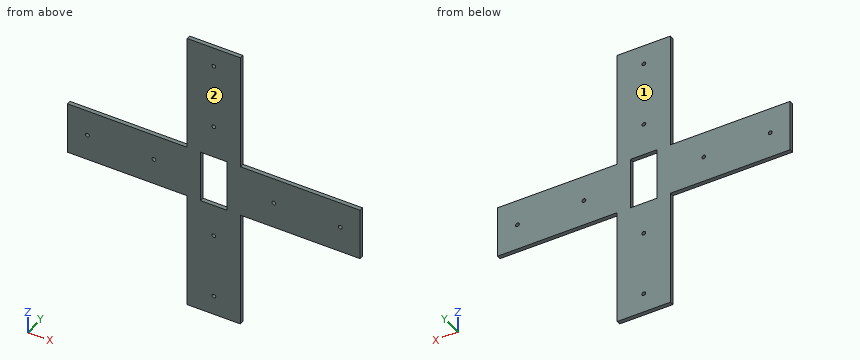
```python
from build123d import *

# Parameters (mm, degrees)
SKETCH1_R           = 1.45
SKETCH1_W           = 20.1
SKETCH1_H           = 40.1
BOSS_EXTRUDE1_DEPTH = 3


with BuildPart() as part:
    # Sketch1 → Boss-Extrude1 (new body)
    with BuildSketch(Plane(origin=(0, 0, 0), x_dir=(1, 0, 0), z_dir=(0, 1, 0))):
        Polygon((-20, 110), (20, 110), (20, 20), (110, 20), (110, -20), (20, -20), (20, -110), (-20, -110), (-20, -20), (-110, -20), (-110, 20), (-20, 20), align=None)
        with Locations(Location((45, 0, 0), (0, 0, 270))):
            Circle(SKETCH1_R, mode=Mode.SUBTRACT)
        with Locations(Location((95, 0, 0), (0, 0, 270))):
            Circle(SKETCH1_R, mode=Mode.SUBTRACT)
        with Locations(Location((-95, 0, 0), (0, 0, 270))):
            Circle(SKETCH1_R, mode=Mode.SUBTRACT)
        with Locations(Location((-45, 0, 0), (0, 0, 270))):
            Circle(SKETCH1_R, mode=Mode.SUBTRACT)
        with Locations(Location((0, 95, 0), (0, 0, 270))):
            Circle(SKETCH1_R, mode=Mode.SUBTRACT)
        with Locations(Location((0, 45, 0), (0, 0, 270))):
            Circle(SKETCH1_R, mode=Mode.SUBTRACT)
        with Locations(Location((0, -45, 0), (0, 0, 270))):
            Circle(SKETCH1_R, mode=Mode.SUBTRACT)
        with Locations(Location((0, -95, 0), (0, 0, 270))):
            Circle(SKETCH1_R, mode=Mode.SUBTRACT)
        Rectangle(SKETCH1_W, SKETCH1_H, mode=Mode.SUBTRACT)
    extrude(amount=BOSS_EXTRUDE1_DEPTH)


solid = part.part
```
Source: CAD feature listing. Evaluate the final solid. Frame: model axes, mm. Face numbers are marked on the shaded views. Give positions to 0.01 mm unless a question says otherwise; leave off trailing zeros. Order: outer loops, then holes, each group sorted by start corner. A loop starts at its lowest first (then second) coordinate and runs counter-clockwise, first axis right, second up.
(1) Section query A-A (y = 0.45). State how many separate pieces and enclosed holes the cut face has, plus the area to 3 significant figures.
(2) Material intervals for line 1 along X through (y, z) = (2.1, 0); line 2 along X through (y, z) = (1.85, 45), sorted ascending.
(3) Section query B-B (z = -52.5). Return the cut outline in (x, y).
(4) Pull-direction query (Y, two-part tool) for the marked faces 1 and 2; classes: +Y half, -Y half, draft (parallel to the pull), parting line (faces both ways), or undercut.
(5) Contact query for flat-ended pins moving along their axis: P1, Ø4.5, axis at x = 0, z = -45, coming from the +Y side; P2, Ø1.5, axis at y = 1.5, z = -86.5, coming from the -X side; P3, Ø0.9, axis at x = 53.5, y = 2, coming from the -Z side. Output: stop coordinate, or through.
(6) Section query C-C (x = -34). Return the cut outline in (y, z), plus the area to 3 significant figures.
Outcome:
1. separate pieces: 1
1. enclosed holes: 9
1. area: 15,100 mm2
2. line 1: x = -110 to -96.45, -93.55 to -46.45, -43.55 to -10.05, 10.05 to 43.55, 46.45 to 93.55, 96.45 to 110
2. line 2: x = -20 to -1.45, 1.45 to 20
3. outline: (-20, 0) - (20, 0) - (20, 3) - (-20, 3) - close
4. face 1: +Y half
4. face 2: -Y half
5. P1: stops at y = 3
5. P2: stops at x = -20
5. P3: stops at z = -20
6. outline: (0, -20) - (3, -20) - (3, 20) - (0, 20) - close
6. area: 120 mm2
